Input: dimensioned drawing with shaded views. Units: mm. Origin: part minimum x, y, z. A direction names the side the tool comes from. Coordinates: 2 decimals unless noted, no trailing zeros. Order: outer loops, then holes, each group sorted by start corner. A loop starts at its lowest first (then second) coordinate and runs counter-clockwise, first axis right, second up. Notation, with made-up numbers: M -19.75,76.5 L 16.25,76.5 A32 cw 16.25,105.5 Z; hole C 34.5,47.25 d3. An arc over 180 degrees is marked long. Use CSV: the item, a comma, the result in double quotes. Start each with the question number.
1. Pull-direction query (X, two-part tool) for the marked faces 1, 2, 3 and 4; classes: pulls with the +X half, pulls with the -X half, needs draft (parallel to the pull), parting line crosses it, or undercut.
2. Section query C-C on x = 19.75. Return the cut outline in (y, z).
3. Material intervals for line 1 (Y direction, x = 11, z = 0.8); line 2 (Y direction, x = 12, z = 1.75); line 3 (Y direction, x = 12.75, z = 1.75), sorted ascending.
4. First-contact query: P1, Ø1, axis at y = 9.5, z = 10.5, coming from the -X side; P2, Ø4, axis at x = 4.5, z = 4.5, coming from the -Y side; P3, Ø3.5, axis at x = 11, y = 3, coming from the +Z side. Flat tips, straight axial feed; report the tip coordinate or a pass-through.
5. Set-up query: the marked faces 5 and 6. Return all of +Z, -Z, +X, -X, +Y, -Y with unobstructed straight access to the full face (end or side cutting, diameter ignored); none if empty.
6. Section query A-A on y = 11. Return the cut outline in (x, z).
7. Section query D-D on y = 3. Return the cut outline in (x, z), and give its area (3 significant figures).
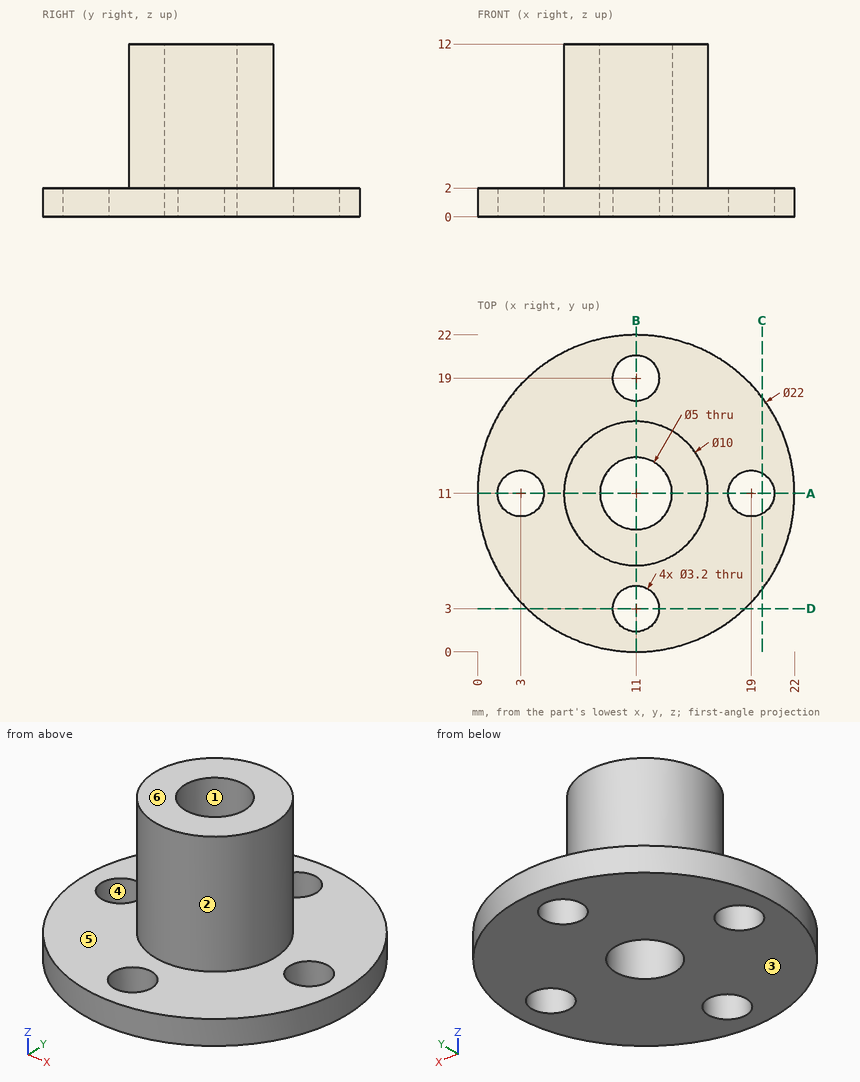
Results list:
1,face 1,"undercut"
1,face 2,"parting line crosses it"
1,face 3,"needs draft"
1,face 4,"undercut"
2,outline,"M 4.33,0 L 9.59,0 L 9.59,2 L 4.33,2 Z; M 12.41,0 L 17.67,0 L 17.67,2 L 12.41,2 Z"
3,line 1,"y = 0 to 1.4, 4.6 to 8.5, 13.5 to 17.4, 20.6 to 22"
3,line 2,"y = 0.05 to 1.75, 4.25 to 8.71, 13.29 to 17.75, 20.25 to 21.95"
3,line 3,"y = 0.14 to 9.21, 12.79 to 21.86"
4,P1,"stops at x = 6.1"
4,P2,"stops at y = 8.82"
4,P3,"stops at z = 2"
5,face 5,"+Z"
5,face 6,"+Z, +X, -X, +Y, -Y"
6,outline,"M 0,0 L 1.4,0 L 1.4,2 L 0,2 Z; M 4.6,0 L 8.5,0 L 8.5,12 L 6,12 L 6,2 L 4.6,2 Z; M 13.5,0 L 17.4,0 L 17.4,2 L 16,2 L 16,12 L 13.5,12 Z; M 20.6,0 L 22,0 L 22,2 L 20.6,2 Z"
7,outline,"M 3.45,0 L 9.4,0 L 9.4,2 L 3.45,2 Z; M 12.6,0 L 18.55,0 L 18.55,2 L 12.6,2 Z"
7,area,"23.8 mm²"
